Verification items for the finished model (mm, model axes). Round coordinates to 2 decimals unless told otherwise and drop trailing zeros. Order: outer loops, then holes, each group sorted by start corner. A loop starts at its lowest first (then second) coordinate and runs counter-clockwise, first axis right, second up. Notation, with made-up numbers: M -17,64 L 5,64 A19 cw 5,70 Z; hole C -11,16.25 d3. An arc over 180 degrees is marked long. Use CSV: the item, a comma, the result in double quotes. Start each with the question number.
Q1. Sectioned sample at C-C (x = 43). Enter the section's corners in (y, z).
Q2. Scan lines: line 1 (Z direction, x = -20, y = -10.5); line 2 (X direction, y = -7.75, z = 15); line 3 (Z direction, x = -46, y = -15.5). Record each from-to range of solid material in increasing order.
Q3. Mould release check, pull along X, two halves, no side actions. Record for faces 1 (the face through (55.51, -12.52, 22.13)), 2 (the face through (-3, 0, 18)), 3 (the face through (-18.206, -12.593, 11.179)), 4 (the face through (-47.152, -4.762, 7.218)): +X half, -X half, draft (parallel to the pull), parting line (faces both ways), or undercut.
Q4. Sectioned sample at D-D (z = 43.5). Enter the section's corners in (x, y), and give its area (3 significant figures).
Q5. Sectioned sample at B-B (y = -9). Enter the section's corners in (x, z).
Q6. Sectioned sample at A-A (y = -24). Enter the section's corners in (x, z), and give its area (3 significant figures).
Q7. Gauge pin test, flat ends, axial feed: pin 1 Ø1.5 at (x, y) = (-1, -19.5) entering from -Z; pin 2 Ø6 at (x, y) = (-11, -8) entering from -Z; pin 3 Ø5 at (x, z) = (-51, 13.5) entering from +Y; pin 4 Ø2 at (x, z) = (-1, 24.5) entering from +Y. Record the tip position at first contact, or that the pin passes through.
```python
from build123d import *

# Parameters (mm, degrees)
F0_R     = 16.708359
F1_DEPTH = 25.4
F2_SIZE  = 5.08
F3_SIZE  = 5.08


with BuildPart() as f1:
    # F0 (on Front) → F1 (new body)
    with BuildSketch(Plane.XZ):
        with BuildLine():
            ThreePointArc((-24.523889, -12.243737), (-8.494482, -0.883461), (-2.350032, 17.777823))
            ThreePointArc((-2.350032, 17.777823), (-8.596971, 36.577077), (-24.852983, 47.898664))
            ThreePointArc((-24.852983, 47.898664), (-65.170116, 17.605951), (-24.523889, -12.243737))
        make_face()
        with Locations((-33.640571, 17.577954)):
            Circle(F0_R, mode=Mode.SUBTRACT)
        with BuildLine():
            ThreePointArc((-24.852983, 47.898664), (-8.596971, 36.577077), (-2.350032, 17.777823))
            ThreePointArc((-2.350032, 17.777823), (-8.494482, -0.883461), (-24.523889, -12.243737))
            Line((-24.523889, -12.243737), (37.955624, 1.879685))
            ThreePointArc((37.955624, 1.879685), (18.047037, 17.790268), (37.955624, 33.70085))
            Line((37.955624, 33.70085), (-24.852983, 47.898664))
        make_face()
        with BuildLine():
            ThreePointArc((49.022596, 24.936072), (44.486406, 30.577711), (37.955624, 33.70085))
            ThreePointArc((37.955624, 33.70085), (18.047037, 17.790268), (37.955624, 1.879685))
            ThreePointArc((37.955624, 1.879685), (44.90086, 5.342284), (49.460027, 11.622401))
            ThreePointArc((49.460027, 11.622401), (50.365449, 14.64745), (50.671074, 17.790268))
            ThreePointArc((50.671074, 17.790268), (50.253612, 21.45701), (49.022596, 24.936072))
        make_face()
        with BuildLine():
            Line((61.825909, 19.396365), (49.022596, 24.936072))
            ThreePointArc((49.022596, 24.936072), (50.253612, 21.45701), (50.671074, 17.790268))
            ThreePointArc((50.671074, 17.790268), (50.365449, 14.64745), (49.460027, 11.622401))
            Line((49.460027, 11.622401), (61.825909, 19.396365))
        make_face()
    extrude(amount=F1_DEPTH)

    # F2
    f2_edges = [f1.edges().sort_by_distance(p)[0] for p in [
        (-50.34893, -25.4, 17.577954),
    ]]
    chamfer(f2_edges, length=F2_SIZE)

    # F3
    f3_edges = [f1.edges().sort_by_distance(p)[0] for p in [
        (-50.34893, 0, 17.577954),
    ]]
    chamfer(f3_edges, length=F3_SIZE)


solid = f1.part
```
Verdict:
1,outline,"M -25.4,3.95 L 0,3.95 L 0,31.63 L -25.4,31.63 Z"
2,line 1,"z = -11.22 to 7.93, 27.23 to 46.8"
2,line 2,"x = -65.05 to -50.15, -17.13 to 54.83"
2,line 3,"z = -11.15 to 6.33, 28.82 to 46.71"
3,face 1,"+X half"
3,face 2,"draft"
3,face 3,"undercut"
3,face 4,"undercut"
4,outline,"M -51.79,-25.4 L -5.39,-25.4 L -5.39,0 L -51.79,0 Z"
4,area,"1,180 mm²"
5,outline,"M -24.85,47.9 A31.41 ccw long -24.52,-12.24 L 37.96,1.88 A16.31 ccw 49.46,11.62 L 61.83,19.4 L 49.02,24.94 A16.31 ccw 37.96,33.7 Z; hole C -33.64,17.58 d33.42"
6,outline,"M -24.85,47.9 A31.41 ccw long -24.52,-12.24 L 37.96,1.88 A16.31 ccw 49.46,11.62 L 61.83,19.4 L 49.02,24.94 A16.31 ccw 37.96,33.7 Z; hole C -33.64,17.58 d40.78"
6,area,"4,060 mm²"
7,pin 1,"stops at z = -7.1"
7,pin 2,"stops at z = -9.86"
7,pin 3,"stops at y = -1.46"
7,pin 4,"stops at y = 0"
